```python
from build123d import *

# Parameters (mm, degrees)
BOSS_EXTRUDE1_DEPTH   = 6.35
M6X1_0_TAPPED_HOLE1_D = 5
LPATTERN1_COUNT       = 49
LPATTERN1_PITCH       = 10
CUT_EXTRUDE1_REACH    = 8.35
SKETCH5_R             = 2.6


with BuildPart() as part:
    # Sketch1 → Boss-Extrude1 (new body)
    with BuildSketch(Plane(origin=(0, 0, 0), x_dir=(1, 0, 0), z_dir=(0, 1, 0))):
        with BuildLine():
            Line((10, 0), (494, 0))
            ThreePointArc((494, 0), (501.071067812, 2.928932188), (504, 10))
            Line((504, 10), (504, 40))
            ThreePointArc((504, 40), (502.535533906, 43.535533906), (499, 45))
            Line((499, 45), (5, 45))
            ThreePointArc((5, 45), (1.464466094, 43.535533906), (0, 40))
            Line((0, 40), (0, 10))
            ThreePointArc((0, 10), (2.928932188, 2.928932188), (10, 0))
        make_face()
    extrude(amount=BOSS_EXTRUDE1_DEPTH)

    # M6x1.0 Tapped Hole1 (through all)
    with Locations(Plane(origin=(0, 6.35, 0), x_dir=(1, 0, 0), z_dir=(0, 1, 0))):
        with Locations((492, 24.6)):
            m6x1_0_tapped_hole1 = Hole(M6X1_0_TAPPED_HOLE1_D / 2)

    # LPattern1: M6x1.0 Tapped Hole1 ×49
    with Locations(*[(-i * LPATTERN1_PITCH, 0, 0) for i in range(1, LPATTERN1_COUNT)]):
        add(m6x1_0_tapped_hole1, mode=Mode.SUBTRACT)

    # Sketch5 → Cut-Extrude1 (cut, up to next)
    with BuildSketch(Plane(origin=(0, 6.35, 0), x_dir=(1, 0, 0), z_dir=(0, 1, 0)), mode=Mode.PRIVATE) as cut_extrude1_sk1:
        with Locations((10, 10)):
            Circle(SKETCH5_R)
    cut_extrude1_tool1 = extrude(cut_extrude1_sk1.sketch, amount=-CUT_EXTRUDE1_REACH, mode=Mode.PRIVATE) & part.part
    add(cut_extrude1_tool1.solids().sort_by_distance((10, 6.35, -10))[0], mode=Mode.SUBTRACT)
    # Sketch5 → Cut-Extrude1 (cut, up to next)
    with BuildSketch(Plane(origin=(0, 6.35, 0), x_dir=(1, 0, 0), z_dir=(0, 1, 0)), mode=Mode.PRIVATE) as cut_extrude1_sk2:
        with Locations((10, 39.2)):
            Circle(SKETCH5_R)
    cut_extrude1_tool2 = extrude(cut_extrude1_sk2.sketch, amount=-CUT_EXTRUDE1_REACH, mode=Mode.PRIVATE) & part.part
    add(cut_extrude1_tool2.solids().sort_by_distance((10, 6.35, -39.2))[0], mode=Mode.SUBTRACT)
    # Sketch5 → Cut-Extrude1 (cut, up to next)
    with BuildSketch(Plane(origin=(0, 6.35, 0), x_dir=(1, 0, 0), z_dir=(0, 1, 0)), mode=Mode.PRIVATE) as cut_extrude1_sk3:
        with Locations((494, 10)):
            Circle(SKETCH5_R)
    cut_extrude1_tool3 = extrude(cut_extrude1_sk3.sketch, amount=-CUT_EXTRUDE1_REACH, mode=Mode.PRIVATE) & part.part
    add(cut_extrude1_tool3.solids().sort_by_distance((494, 6.35, -10))[0], mode=Mode.SUBTRACT)
    # Sketch5 → Cut-Extrude1 (cut, up to next)
    with BuildSketch(Plane(origin=(0, 6.35, 0), x_dir=(1, 0, 0), z_dir=(0, 1, 0)), mode=Mode.PRIVATE) as cut_extrude1_sk4:
        with Locations((494, 39.2)):
            Circle(SKETCH5_R)
    cut_extrude1_tool4 = extrude(cut_extrude1_sk4.sketch, amount=-CUT_EXTRUDE1_REACH, mode=Mode.PRIVATE) & part.part
    add(cut_extrude1_tool4.solids().sort_by_distance((494, 6.35, -39.2))[0], mode=Mode.SUBTRACT)
    # Sketch5 → Cut-Extrude1 (cut, up to next)
    with BuildSketch(Plane(origin=(0, 6.35, 0), x_dir=(1, 0, 0), z_dir=(0, 1, 0)), mode=Mode.PRIVATE) as cut_extrude1_sk5:
        with Locations((252, 10)):
            Circle(SKETCH5_R)
    cut_extrude1_tool5 = extrude(cut_extrude1_sk5.sketch, amount=-CUT_EXTRUDE1_REACH, mode=Mode.PRIVATE) & part.part
    add(cut_extrude1_tool5.solids().sort_by_distance((252, 6.35, -10))[0], mode=Mode.SUBTRACT)
    # Sketch5 → Cut-Extrude1 (cut, up to next)
    with BuildSketch(Plane(origin=(0, 6.35, 0), x_dir=(1, 0, 0), z_dir=(0, 1, 0)), mode=Mode.PRIVATE) as cut_extrude1_sk6:
        with Locations((252, 39.2)):
            Circle(SKETCH5_R)
    cut_extrude1_tool6 = extrude(cut_extrude1_sk6.sketch, amount=-CUT_EXTRUDE1_REACH, mode=Mode.PRIVATE) & part.part
    add(cut_extrude1_tool6.solids().sort_by_distance((252, 6.35, -39.2))[0], mode=Mode.SUBTRACT)


solid = part.part
```
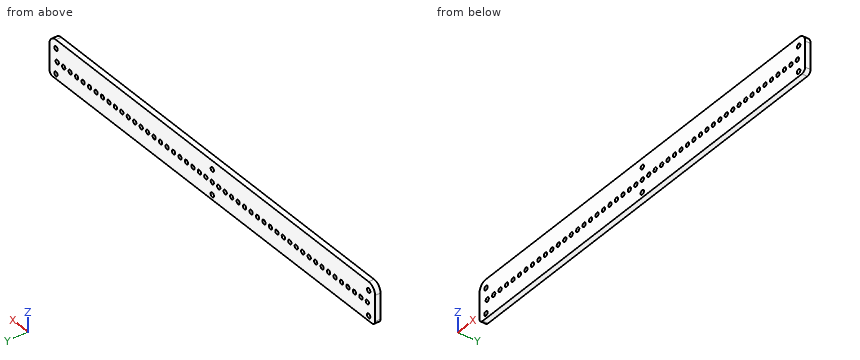
CAD build for the part. Positions are in the model's coordinates, mm. Coordinates: 2 decimals unless noted, no trailing zeros. Return JSON: item names as keys, results as strings.
1. Probe L1, parallel to Z at x = 402, y = 3; L2, parallel to X at y = 1.25, z = -39; L3, parallel to Z at x = 252, y = 3. List the from-to ranges inside material, lowest first. Write a range as from..to.
Result:
{"L1": "z = -45..-27.1, -22.1..0", "L2": "x = 0..7.41, 12.59..249.41, 254.59..491.41, 496.59..504", "L3": "z = -45..-41.8, -36.6..-27.1, -22.1..-12.6, -7.4..0"}
2. Band-saw the part on A-A (y = 1.75). State how many separate pieces and enclosed holes the cut face has, and give its area (3 significant figures).
Result:
{"separate pieces": "1", "enclosed holes": "55", "area": "21,500 mm2"}
3. Drop a flat-ended pin along its axis: pin 1 (3 mm diameter, centred on x = 62, z = -24.6, fed in from -Y). Give the stop position or say it passes through.
Result:
{"pin 1": "passes through"}
